Drawing for the job (mm, zero at the part's lowest x, y, z). Round coordinates to 2 decimals unless told otherwise and drop trailing zeros. Write each loop counter-clockwise with the first axis right and the second up, starting at its lowest first coordinate (ties: lowest second). Pieces come first, ordered by that corner, then holes.
Item 1: Wall check: probe 1 along X at (y, z) = (2.85, 69); probe 2 along X at (y, z) = (2.6, 25) (3 decimals); probe 3 along Z at (x, y) = (20, 2.8). Give the ranges that are in metal, low to high.
Item 2: Band-saw the part on C-C, the plane y = 1.8. Write the cut outline in (x, z) (3 decimals), then the cut area to 3 significant figures.
Item 3: Drop flat-ended pins along their axis: pin 1 Ø1.5 at (y, z) = (1, 22.5) entering from -X; pin 2 Ø16.5 at (x, z) = (22, 25.5) entering from +Y; pin 3 Ø2.5 at (x, z) = (10, 69) entering from -Y. Give the stop position or say it passes through.
Item 4: Band-saw the part on D-D, the plane x = 25. Write the cut outline in (y, z) (3 decimals), then the cut area to 3 significant figures.
Item 5: Band-saw the part on B-B, the plane z = 69. Write the cut outline in (x, y), then the cut area to 3 significant figures.
Item 6: Band-saw the part on A-A, the plane x = 40. Write the cut outline in (y, z).
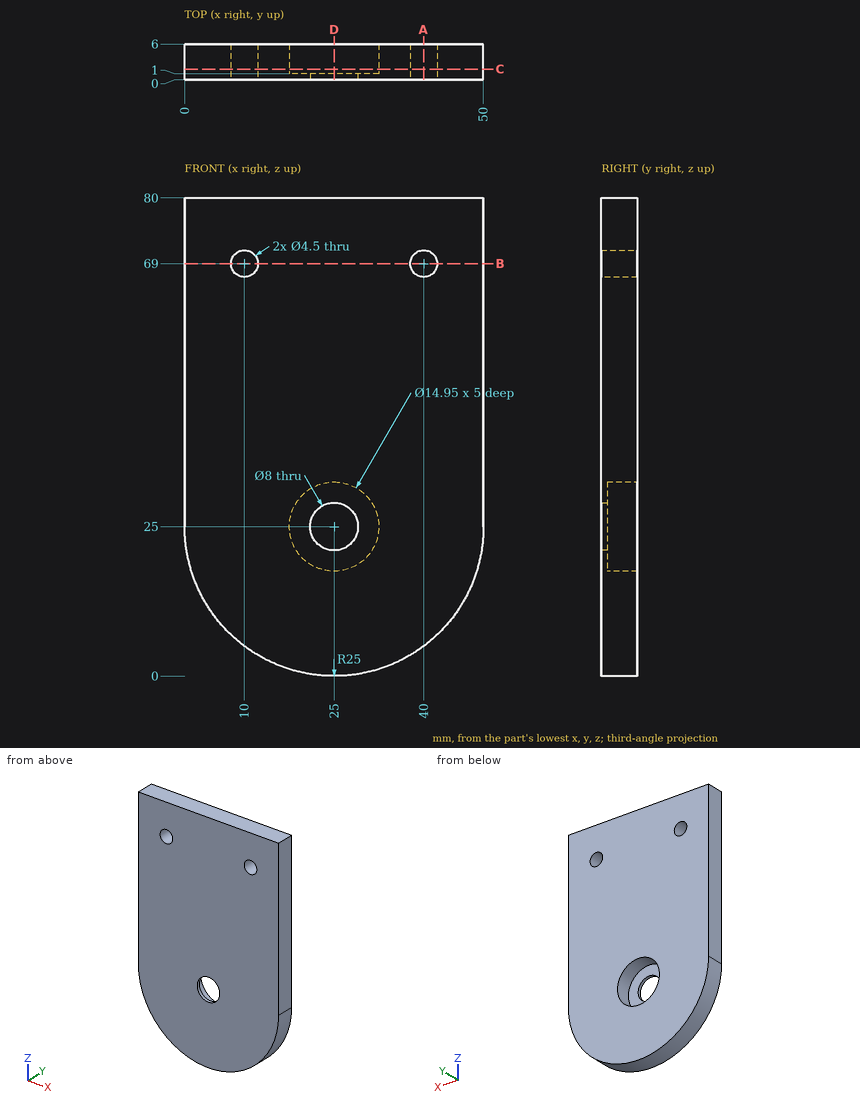
Results:
1. probe 1: x = 0 to 7.75, 12.25 to 37.75, 42.25 to 50
1. probe 2: x = 0 to 17.525, 32.475 to 50
1. probe 3: z = 0.51 to 19.44, 30.56 to 80
2. outline: (0, 25) arc R25 ccw to (50, 25) - (50, 80) - (0, 80) - close; hole circle Ø4.5 at (10, 69); hole circle Ø14.95 at (25, 25); hole circle Ø4.5 at (40, 69)
2. area: 3,520 mm2
3. pin 1: stops at x = 0.06
3. pin 2: stops at y = 6
3. pin 3: passes through
4. outline: (0, 0) - (6, 0) - (6, 17.525) - (1, 17.525) - (1, 21) - (0, 21) - close; (0, 29) - (1, 29) - (1, 32.475) - (6, 32.475) - (6, 80) - (0, 80) - close
4. area: 397 mm2
5. outline: (0, 0) - (7.75, 0) - (7.75, 6) - (0, 6) - close; (12.25, 0) - (37.75, 0) - (37.75, 6) - (12.25, 6) - close; (42.25, 0) - (50, 0) - (50, 6) - (42.25, 6) - close
5. area: 246 mm2
6. outline: (0, 5) - (6, 5) - (6, 66.75) - (0, 66.75) - close; (0, 71.25) - (6, 71.25) - (6, 80) - (0, 80) - close
